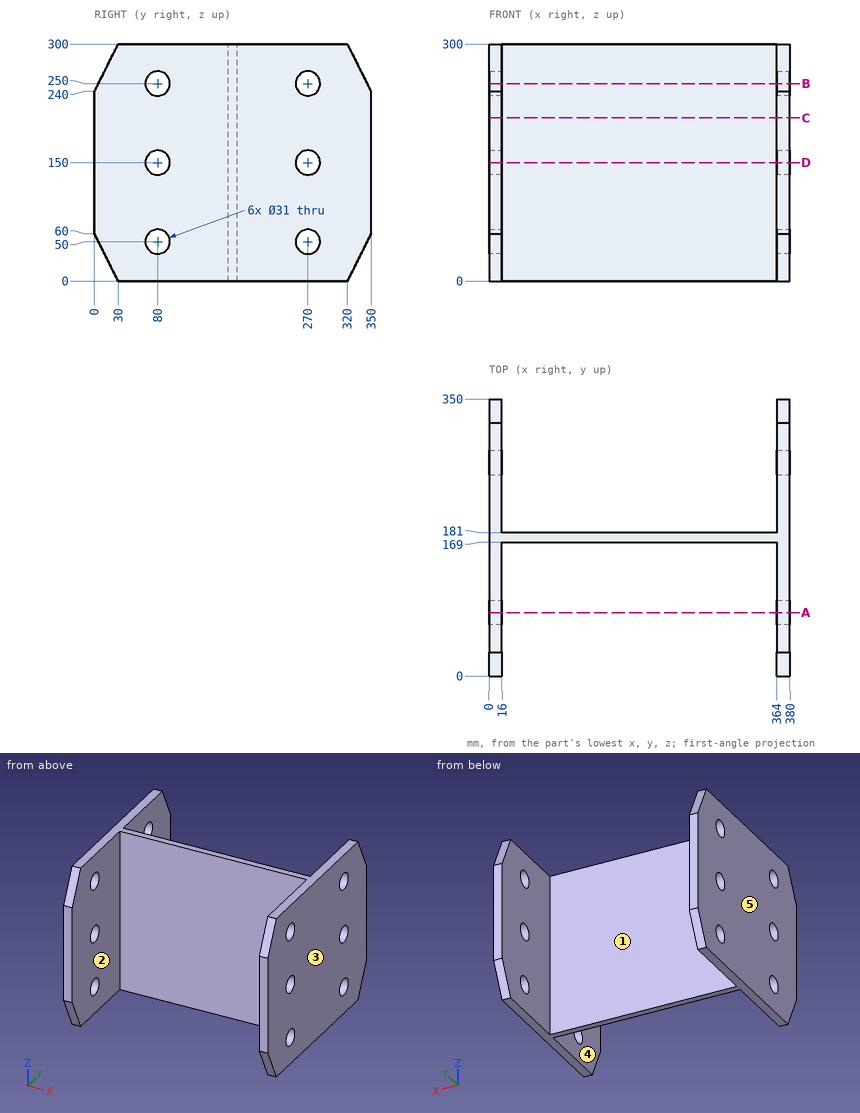
Input: dimensioned drawing with shaded views. Units: mm. Origin: part minimum x, y, z. A direction names the side the tool comes from. Coordinates: 2 decimals unless noted, no trailing zeros. Loops run counter-clockwise (first coordinate to the right, second up) from the corner with the lowest first, then second, coordinate; pieces in that order, holes last. Notation, with made-up numbers: (-26, 75) - (18, 75) arc R12 cw to (18, 79) - close; hole circle Ø8 at (83, -32). An arc over 180 degrees is marked (long way). One line per question, with ' | ' between items. Start each with the question number.
(1) Draft query along X for the marked faces 3, 4 and 5. Return one class per face: +X half, -X half, draft (parallel to the pull), parting line (faces both ways), or undercut.
(2) Cut plane C-C on z = 206.5. Output: boundary loops of the cut face in (x, y).
(3) Cut plane A-A on y = 80. Count the separate pieces of the cut face and the enclosed holes in it, and give its area (3 significant figures).
(4) Cut plane D-D on z = 150. Output: boundary loops of the cut face in (x, y), and give its area (3 significant figures).
(5) Cut plane B-B on z = 250. Output: boundary loops of the cut face in (x, y).
(6) First-contact query: pin 1 (2 mm diameter, centred on x = 80, z = 184, fed in from -Y); pin 2 (18.5 mm diameter, centred on y = 80, z = 50, fed in from +X). Flat tips, straight axial feed; report the tip coordinate or a pass-through.
(7) Reachability of the marked faces 1 and 2 from +Z, -Z, +X, -X, +Y, -Y: full face, straight path, thin tool, end or side. Return the list, or none.
(8) Ray query, L1, parallel to X at y = 239, z = 226.5; L2, parallel to Y at x = 258, z = 166. Return the intervals inside material, ascending. Write a range as from..to.
Here are the results:
1) face 3: +X half | face 4: undercut | face 5: -X half
2) outline: (0, 0) - (16, 0) - (16, 169) - (364, 169) - (364, 0) - (380, 0) - (380, 350) - (364, 350) - (364, 181) - (16, 181) - (16, 350) - (0, 350) - close
3) separate pieces: 8 | enclosed holes: 0 | area: 6,620 mm²
4) outline: (0, 0) - (16, 0) - (16, 64.5) - (0, 64.5) - close; (0, 95.5) - (16, 95.5) - (16, 169) - (364, 169) - (364, 95.5) - (380, 95.5) - (380, 254.5) - (364, 254.5) - (364, 181) - (16, 181) - (16, 254.5) - (0, 254.5) - close; (0, 285.5) - (16, 285.5) - (16, 350) - (0, 350) - close; (364, 0) - (380, 0) - (380, 64.5) - (364, 64.5) - close; (364, 285.5) - (380, 285.5) - (380, 350) - (364, 350) - close | area: 13,400 mm²
5) outline: (0, 5) - (16, 5) - (16, 64.5) - (0, 64.5) - close; (0, 95.5) - (16, 95.5) - (16, 169) - (364, 169) - (364, 95.5) - (380, 95.5) - (380, 254.5) - (364, 254.5) - (364, 181) - (16, 181) - (16, 254.5) - (0, 254.5) - close; (0, 285.5) - (16, 285.5) - (16, 345) - (0, 345) - close; (364, 5) - (380, 5) - (380, 64.5) - (364, 64.5) - close; (364, 285.5) - (380, 285.5) - (380, 345) - (364, 345) - close
6) pin 1: y = 169 | pin 2: through
7) face 1: +Z, -Z, +Y | face 2: +Z, -Z, -Y
8) L1: 0..16, 364..380 | L2: 169..181
